Here's how the part is built. I have some questions about the finished solid (model axes, mm). A direction names the side the tool comes from. Give positions to 0.01 mm unless a question says otherwise; leave off trailing zeros. Write each loop counter-clockwise with the first axis right and the second up, starting at its lowest first coordinate (ties: lowest second). Pieces come first, ordered by that corner, then holes. Notation, with made-up numbers: (3.25, 33.25) -> (34.25, 33.25) arc R23 cw to (34.25, 72.25) -> close; hole circle Ø3 at (63, 21). An arc over 180 degrees is marked (long way). Use CSV: the item, a comma, the result in double quotes. Start each with the question number.
(1) I need wall thicknesses on L1, parallel to X at y = 111, z = 40; L2, parallel to X at y = 126, z = 81.5; L3, parallel to Y at x = 63, z = 92.5. Which ranges of each line are inside material? Lowest first, please. Write a range as [from, to].
(2) Suppose I cut it at C-C on z = 73. List the corners of the cut face in (x, y) for me.
(3) Suppose I cut it at D-D on z = 98.5. List the corners of the cut face in (x, y) for me, plus the area to 3 significant figures.
(4) For pin 1 Ø6 at (y, z) = (150.5, 72.5) entering from +X, with a flat end and sliding along its axis, tell me the tip position at first contact or that it passes through.
(5) Which directions (+Z, -Z, +X, -X, +Y, -Y) give clear straight access to the entire face, cutting with the end or side of a thin tool? Please do faces 4 (the flat face through (2.54, 88, 38)), 5 (the flat face through (135, 177.8, 63)), 6 (the flat face through (235, 175.26, 63)).
(6) Suppose I cut it at B-B on y = 140.5. List the corners of the cut face in (x, z) for me, plus the area to 3 significant figures.
(7) Suppose I cut it at A-A on x = 204.5. List the corners of the cut face in (y, z) for me.
(8) If we mould it in two halves opening along X, with no side actions, what happens to faces 1 (the flat face through (2.085, 88.485, 77.022)), 2 (the flat face through (129.54, 88, 63)), 3 (the flat face through (131, 89, 127))? For each: pulls with the +X half, pulls with the -X half, needs draft (parallel to the pull), parting line crosses it, or undercut.
from build123d import *

# Parameters (mm, degrees)
F0_W     = 273.05
F0_H     = 177.8
F0_W_2   = 267.97
F0_H_2   = 172.72
F1_DEPTH = 127
F2_W     = 2.54
F2_H     = 172.72
F3_DEPTH = 127
F5_DEPTH = 177.801
F6_W     = 172.72
F6_H     = 127
F7_DEPTH = 25.4


with BuildPart() as f1:
    # F0 (on Top) → F1 (new body)
    with BuildSketch(Plane.XY):
        with Locations((136.525, 88.9)):
            Rectangle(F0_W, F0_H)
        with Locations((136.525, 88.9)):
            Rectangle(F0_W_2, F0_H_2, mode=Mode.SUBTRACT)
    extrude(amount=F1_DEPTH)

    # F2 (on Top) → F3 (join)
    with BuildSketch(Plane.XY):
        with Locations((67.31, 88.9)):
            Rectangle(F2_W, F2_H)
        with Locations((130.81, 88.9)):
            Rectangle(F2_W, F2_H)
        with Locations((194.31, 88.9)):
            Rectangle(F2_W, F2_H)
    extrude(amount=F3_DEPTH)

    # F4 (on face) → F5 (cut, through all)
    with BuildSketch(Plane.XZ):
        Polygon((0, 76.2), (128.840938, 127), (0, 127), align=None)
    extrude(amount=-F5_DEPTH, mode=Mode.SUBTRACT)

    # F6 (on face) → F7 (cut)
    with BuildSketch(Plane.YZ.offset(273.05)):
        with Locations((88.9, 63.5)):
            Rectangle(F6_W, F6_H)
    extrude(amount=-F7_DEPTH, mode=Mode.SUBTRACT)


solid = f1.part
Geometry says:
1,L1,"[0, 2.54], [66.04, 68.58], [129.54, 132.08], [193.04, 195.58]"
1,L2,"[66.04, 68.58], [129.54, 132.08], [193.04, 195.58]"
1,L3,"[0, 2.54], [175.26, 177.8]"
2,outline,"(0, 0) -> (273.05, 0) -> (273.05, 2.54) -> (195.58, 2.54) -> (195.58, 175.26) -> (273.05, 175.26) -> (273.05, 177.8) -> (0, 177.8) -> close; hole (2.54, 2.54) -> (66.04, 2.54) -> (66.04, 175.26) -> (2.54, 175.26) -> close; hole (68.58, 2.54) -> (129.54, 2.54) -> (129.54, 175.26) -> (68.58, 175.26) -> close; hole (132.08, 2.54) -> (193.04, 2.54) -> (193.04, 175.26) -> (132.08, 175.26) -> close"
3,outline,"(56.56, 0) -> (273.05, 0) -> (273.05, 2.54) -> (195.58, 2.54) -> (195.58, 175.26) -> (273.05, 175.26) -> (273.05, 177.8) -> (56.56, 177.8) -> (56.56, 175.26) -> (66.04, 175.26) -> (66.04, 2.54) -> (56.56, 2.54) -> close; hole (68.58, 2.54) -> (129.54, 2.54) -> (129.54, 175.26) -> (68.58, 175.26) -> close; hole (132.08, 2.54) -> (193.04, 2.54) -> (193.04, 175.26) -> (132.08, 175.26) -> close"
3,area,"2,420 mm²"
4,pin 1,"x = 195.58"
5,face 4,"+Z, -Z"
5,face 5,"+Z, -Z, +X, -X, +Y"
5,face 6,"+Z, -Z, +X"
6,outline,"(0, 0) -> (2.54, 0) -> (2.54, 77.2) -> (0, 76.2) -> close; (66.04, 0) -> (68.58, 0) -> (68.58, 103.24) -> (66.04, 102.24) -> close; (129.54, 0) -> (132.08, 0) -> (132.08, 127) -> (129.54, 127) -> close; (193.04, 0) -> (195.58, 0) -> (195.58, 127) -> (193.04, 127) -> close"
6,area,"1,100 mm²"
7,outline,"(0, 0) -> (2.54, 0) -> (2.54, 127) -> (0, 127) -> close; (175.26, 0) -> (177.8, 0) -> (177.8, 127) -> (175.26, 127) -> close"
8,face 1,"pulls with the -X half"
8,face 2,"undercut"
8,face 3,"needs draft"
